from build123d import *

# Parameters (mm, degrees)
SKETCH_1_W          = 33
SKETCH_1_H          = 33
EXTRUDE_1_DEPTH     = 2
SKETCH_2_R          = 1.5
CUT_EXTRUDE_1_DEPTH = 24.420076857
FILLET_1_R          = 5
SKETCH_3_R          = 11
CUT_EXTRUDE_2_DEPTH = 24.420076857


with BuildPart() as part:
    # 草图1 → 凸台-拉伸1 (new body)
    with BuildSketch(Plane.XY):
        Rectangle(SKETCH_1_W, SKETCH_1_H)
    extrude(amount=EXTRUDE_1_DEPTH)

    # 草图2 → 切除-拉伸1 (cut, through all)
    with BuildSketch(Plane.XY.offset(2)):
        with Locations((-12.5, 12.5)):
            Circle(SKETCH_2_R)
        with Locations((-12.5, -12.5)):
            Circle(SKETCH_2_R)
        with Locations((12.5, -12.5)):
            Circle(SKETCH_2_R)
        with Locations((12.5, 12.5)):
            Circle(SKETCH_2_R)
    extrude(amount=-CUT_EXTRUDE_1_DEPTH, mode=Mode.SUBTRACT)

    # 圆角1
    fillet_1_edges = [part.edges().sort_by_distance(p)[0] for p in [
        (16.5, -16.5, 1),
        (-16.5, -16.5, 1),
        (-16.5, 16.5, 1),
        (16.5, 16.5, 1),
    ]]
    fillet(fillet_1_edges, radius=FILLET_1_R)

    # 草图3 → 切除-拉伸2 (cut, through all)
    with BuildSketch(Plane.XY.offset(2)):
        Circle(SKETCH_3_R)
    extrude(amount=-CUT_EXTRUDE_2_DEPTH, mode=Mode.SUBTRACT)


solid = part.part
Here's how the part is built. I have some questions about the finished solid (model axes, mm). Round coordinates to 2 decimals unless told otherwise and drop trailing zeros. Loops run counter-clockwise (first coordinate to the right, second up) from the corner with the lowest first, then second, coordinate; pieces in that order, holes last. Notation, with made-up numbers: (-39.75, -23) - (-33.75, -23) arc R16 ccw to (-33.75, -7) - close; hole circle Ø7 at (58.5, -9.5). An arc over 180 degrees is marked (long way). One line per question, with ' | ' between items. Start each with the question number.
Q1. I want a section at D-D (y = -12.5). Write out the boundary of the cut face in (x, z).
Q2. I want a section at A-A (z = 1.6). Write out the boundary of the cut face in (x, y).
Q3. We'd pull the mould along Y, two halves only. Please class faces 1 (the cylindrical face through (-2.38, -10.74, 1.01)), 2 (the cylindrical face through (-15.07, -15, 1.01)), 3 (the flat face through (-0.2, 11.2, 2)): +Y half, -Y half, draft (parallel to the pull), parting line (faces both ways), or undercut.
Q4. I want a section at B-B (y = 5). Write out the boundary of the cut face in (x, z).
Q5. Will this pin go through, and if not, where does the flat tip stop? pin 1 (10 mm diameter, centred on x = -4, y = -7, fed in from +Z).
Q6. Please list where these lines run through material, in increasing order: line 1 (Y direction, x = 0, z = 0.5); line 2 (Y direction, x = -12.5, z = 0.8); line 3 (Y direction, x = -13.5, z = 1.4). Write a range as [from, to].
Q7. I want a section at C-C (x = 0.5). Write out the boundary of the cut face in (y, z).
Response values:
1) outline: (-16.4, 0) - (-14, 0) - (-14, 2) - (-16.4, 2) - close; (-11, 0) - (11, 0) - (11, 2) - (-11, 2) - close; (14, 0) - (16.4, 0) - (16.4, 2) - (14, 2) - close
2) outline: (-16.5, -11.5) arc R5 ccw to (-11.5, -16.5) - (11.5, -16.5) arc R5 ccw to (16.5, -11.5) - (16.5, 11.5) arc R5 ccw to (11.5, 16.5) - (-11.5, 16.5) arc R5 ccw to (-16.5, 11.5) - close; hole circle Ø3 at (-12.5, -12.5); hole circle Ø3 at (-12.5, 12.5); hole circle Ø22 at (0, 0); hole circle Ø3 at (12.5, -12.5); hole circle Ø3 at (12.5, 12.5)
3) face 1: undercut | face 2: -Y half | face 3: draft
4) outline: (-16.5, 0) - (-9.8, 0) - (-9.8, 2) - (-16.5, 2) - close; (9.8, 0) - (16.5, 0) - (16.5, 2) - (9.8, 2) - close
5) pin 1: stops at z = 2
6) line 1: y = [-16.5, -11], [11, 16.5] | line 2: y = [-16.4, -14], [-11, 11], [14, 16.4] | line 3: y = [-16.08, -13.62], [-11.38, 11.38], [13.62, 16.08]
7) outline: (-16.5, 0) - (-10.99, 0) - (-10.99, 2) - (-16.5, 2) - close; (10.99, 0) - (16.5, 0) - (16.5, 2) - (10.99, 2) - close
